from build123d import *

# Parameters (mm, degrees)
SKETCH_1_W          = 60
SKETCH_1_H          = 20
EXTRUDE_1_DEPTH     = 3
EXTRUDE_2_DEPTH     = 3
EXTRUDE_START       = -3
EXTRUDE_3_DEPTH     = 3
SKETCH_4_R          = 4
SKETCH_4_R_2        = 0.75
CUT_EXTRUDE_1_DEPTH = 70.202601107
SKETCH_5_R          = 4
SKETCH_5_R_2        = 0.75
CUT_EXTRUDE_2_DEPTH = 3
CHAMFER_1_SIZE      = 3


with BuildPart() as part:
    # 草图1 → 凸台-拉伸1 (new body)
    with BuildSketch(Plane(origin=(0, 0, 0), x_dir=(1, 0, 0), z_dir=(0, 1, 0))):
        Rectangle(SKETCH_1_W, SKETCH_1_H)
    extrude(amount=EXTRUDE_1_DEPTH)

    # 草图2 → 凸台-拉伸2 (add)
    with BuildSketch(Plane(origin=(30, 0, 0), x_dir=(0, 0, -1), z_dir=(1, 0, 0))):
        with BuildLine():
            Line((-10, 3), (-10, 23))
            ThreePointArc((-10, 23), (0, 33), (10, 23))
            Line((10, 23), (10, 3))
            Line((10, 3), (-10, 3))
        make_face()
    extrude(amount=-EXTRUDE_2_DEPTH)

    # 草图3 → 凸台-拉伸3 (add)
    with BuildSketch(Plane.ZY.offset(30).offset(EXTRUDE_START)):
        with BuildLine():
            Line((-10, 3), (10, 3))
            Line((10, 3), (10, 23))
            ThreePointArc((10, 23), (0, 33), (-10, 23))
            Line((-10, 23), (-10, 3))
        make_face()
    extrude(amount=EXTRUDE_3_DEPTH)

    # 草图4 → 切除-拉伸1 (cut, through all)
    with BuildSketch(Plane.ZY.offset(30)):
        with Locations((0, 23)):
            Circle(SKETCH_4_R)
        with Locations((0, 29.8)):
            Circle(SKETCH_4_R_2)
        with Locations((6.8, 23)):
            Circle(SKETCH_4_R_2)
        with Locations((0, 16.2)):
            Circle(SKETCH_4_R_2)
        with Locations((-6.8, 23)):
            Circle(SKETCH_4_R_2)
    extrude(amount=-CUT_EXTRUDE_1_DEPTH, mode=Mode.SUBTRACT)

    # 草图5 → 切除-拉伸2 (cut)
    with BuildSketch(Plane(origin=(0, 3, 0), x_dir=(1, 0, 0), z_dir=(0, 1, 0))):
        with Locations(Location((0, 0, 0), (0, 0, 270))):
            Circle(SKETCH_5_R)
        with Locations(Location((0, 6.8, 0), (0, 0, 270))):
            Circle(SKETCH_5_R_2)
        with Locations(Location((6.8, 0, 0), (0, 0, 270))):
            Circle(SKETCH_5_R_2)
        with Locations(Location((0, -6.8, 0), (0, 0, 270))):
            Circle(SKETCH_5_R_2)
        with Locations(Location((-6.8, 0, 0), (0, 0, 270))):
            Circle(SKETCH_5_R_2)
    extrude(amount=-CUT_EXTRUDE_2_DEPTH, mode=Mode.SUBTRACT)

    # 倒角1
    chamfer_1_edges = [part.edges().sort_by_distance(p)[0] for p in [
        (27, 3, 0),
        (-27, 3, 0),
    ]]
    chamfer(chamfer_1_edges, length=CHAMFER_1_SIZE)


solid = part.part
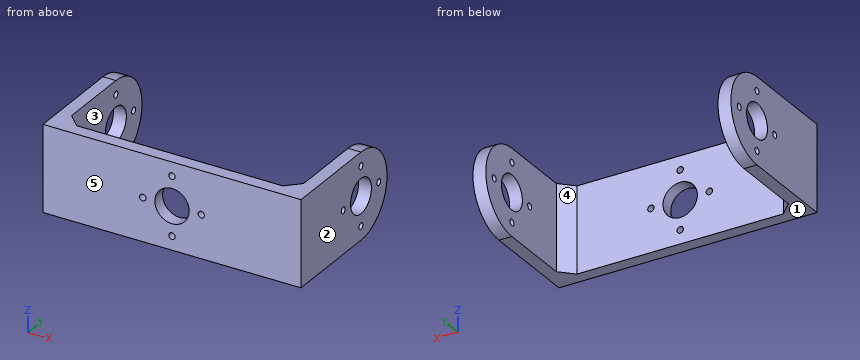
Source: CAD feature listing. Evaluate the final solid. Frame: model axes, mm. Face numbers are marked on the shaded views. A direction names the side the tool comes from. Give positions to 0.01 mm unless a question says otherwise; leave off trailing zeros. Write each loop counter-clockwise with the first axis right and the second up, starting at its lowest first coordinate (ties: lowest second). Pieces come first, ordered by that corner, then holes. Notation, with made-up numbers: (63, 38.5) -> (78, 38.5) arc R24 ccw to (78, 49.5) -> close; hole circle Ø2 at (10.5, 82). An arc over 180 degrees is marked (long way). Return JSON: item names as keys, results as strings. Group by question number.
1. Material intervals for line 1 (Y direction, x = 27.7, z = 0); line 2 (X direction, y = 1.1, z = 0); line 3 (X direction, y = 14, z = -3), sorted ascending. Write a range as from..to.
2. Access query for the marked faces 4 and 5. Directions: +Z, -Z, +X, -X, +Y, -Y. A direction counts if a zero-diameter tool reaches every point of the face in a straight line with its end or side. Return the directions, or none.
3. Section B-B, the plane x = -6.8. Output: boundary loops of the cut face in (y, z).
4. Mould query, pull axis X, two halves, no side actions, for the marked faces 1, 2 and 3. Classes: +X half, -X half, draft (parallel to the pull), parting line (faces both ways), or undercut.
5. Section D-D, the plane z = -6.8. Output: boundary loops of the cut face in (x, y), then the cut area to 3 significant figures.
6. Section C-C, the plane y = 13. Output: boundary loops of the cut face in (x, z), then the cut area to 3 significant figures.
7. Pin query (flat end, axial travel): pin 1 Ø3 at (x, z) = (-19.5, -6.5) entering from +Y. Return the tip coordinate at first contact, or that it passes through.
8. Section A-A, the plane x = 0. Output: boundary loops of the cut face in (y, z).
Determined:
{
 "1": {"line 1": "y = 0..15.45, 16.95..19, 27..29.05, 30.55..33", "line 2": "x = -30..-7.55, -6.05..-4, 4..6.05, 7.55..30", "line 3": "x = -30..-27, 27..30"},
 "2": {"face 4": "+Z, -Z, +Y", "face 5": "+Z, -Z, +X, -X, -Y"},
 "3": {"outline": "(0, -10) -> (3, -10) -> (3, -0.75) -> (0, -0.75) -> close; (0, 0.75) -> (3, 0.75) -> (3, 10) -> (0, 10) -> close"},
 "4": {"face 1": "draft", "face 2": "+X half", "face 3": "undercut"},
 "5": {"outline": "(-30, 0) -> (-0.75, 0) -> (-0.75, 3) -> (-24, 3) -> (-27, 6) -> (-27, 22.25) -> (-30, 22.25) -> close; (-30, 23.75) -> (-27, 23.75) -> (-27, 30.33) -> (-30, 30.33) -> close; (0.75, 0) -> (30, 0) -> (30, 22.25) -> (27, 22.25) -> (27, 6) -> (24, 3) -> (0.75, 3) -> close; (27, 23.75) -> (30, 23.75) -> (30, 30.33) -> (27, 30.33) -> close", "area": "339 mm2"},
 "6": {"outline": "(-30, -10) -> (-27, -10) -> (-27, 10) -> (-30, 10) -> close; (27, -10) -> (30, -10) -> (30, 10) -> (27, 10) -> close", "area": "120 mm2"},
 "7": {"pin 1": "stops at y = 3"},
 "8": {"outline": "(0, -10) -> (3, -10) -> (3, -7.55) -> (0, -7.55) -> close; (0, -6.05) -> (3, -6.05) -> (3, -4) -> (0, -4) -> close; (0, 4) -> (3, 4) -> (3, 6.05) -> (0, 6.05) -> close; (0, 7.55) -> (3, 7.55) -> (3, 10) -> (0, 10) -> close"}
}
